Read the model definition and answer for the solid it produces. Units are mm, in the model's axes. A direction names the side the tool comes from. Round coordinates to 2 decimals unless told otherwise and drop trailing zeros. Order: outer loops, then holes, each group sorted by start corner. A loop starts at its lowest first (then second) coordinate and runs counter-clockwise, first axis right, second up. Notation, with made-up numbers: (81.5, 55.25) -> (85.5, 55.25) arc R14 ccw to (85.5, 80.25) -> close; hole circle Ø7 at (69.25, 86.25). An arc over 180 degrees is marked (long way). Use a Markdown table: item, result. Add a question column.
1. Section D-D, the plane z = 11.25 is taken. Give the vertices of the cut face in (x, y).
2. The mould has two halves that part along Y. Classify faces 5 (the face through (11, -4.25, 8)), 6 (the face through (3.73, -3.8, 1.48)), 7 (the face through (0, -5, 8)): +Y half, -Y half, draft (parallel to the pull), parting line (faces both ways), or undercut.
3. Section A-A, the plane x = 8 is taken. Give the vertices of the cut face in (y, z) (3 decimals).
4. Given pin 1 (1.1 mm diameter, centred on x = 4.5, y = -7, fed in from -Z); pin 2 (0.7 mm diameter, centred on x = 13.5, y = -4.5, fed in from -Z); pin 3 (1 mm diameter, centred on y = -9, z = 6, fed in from +X), each flat-ended and moving along its own axis, determine where each tip first touches the part or whether it passes through.
5. Consider L1, parallel to Y at x = 5.14, z = 1.5; L2, parallel to X at y = -7.63, z = 1.6; L3, parallel to Z at x = 16.9, y = -7.64. Determine where each line is inside the solid, lowest interval first. Write a range as [from, to].
6. Section B-B, the plane x = 12.75 is taken. Give the vertices of the cut face in (y, z), then the cut area to 3 significant figures.
7. Section C-C, the plane y = -5.25 is taken. Give the vertices of the cut face in (x, z), then the cut area to 3 significant figures.
8. For faces 1 (the face through (2, -3.7, 10)), 2 (the face through (13, -2, 9.73)), 3 (the face through (1, -3, 1)), 4 (the face through (13, -5, 13.83)), determine the directions among +Z, -Z, +X, -X, +Y, -Y from which every point of the face is accessible in a straight line to the end or side of a thin tool.
```python
from build123d import *

# Parameters (mm, degrees)
F1_DEPTH  = 10.14
F2_R      = 1.91
F2_W      = 1
F2_H      = 2.7
F3_DEPTH  = 3
F4_W      = 2.5
F4_H      = 3.45
F5_DEPTH  = 5
F6_R      = 1.5
F7_DEPTH  = 2
F9_DEPTH  = 8.95
F11_DEPTH = 8.95
F12_R     = 0.75
F13_DEPTH = 5
F14_R     = 0.75
F15_DEPTH = 5
F16_W     = 9.15
F16_H     = 1.7
F17_DEPTH = 1
F20_DEPTH = 1


with BuildPart() as f1:
    # F0 (on Front) → F1 (new body)
    with BuildSketch(Plane.XZ):
        Polygon((8.4, 15), (0, 15), (0, 0), (8.4, 0), (8.4, 9.23), (17.35, 9.23), (17.35, 13.83), (8.4, 13.83), align=None)
    extrude(amount=F1_DEPTH)

    # F2 (on face) → F3 (cut)
    with BuildSketch(Plane(origin=(0, 0, 0), x_dir=(1, 0, 0), z_dir=(0, 0, -1))):
        with Locations((5.14, 2.51)):
            Circle(F2_R)
        with Locations((5.14, 7.63)):
            Circle(F2_R)
        with Locations((1.5, 2.55)):
            Rectangle(F2_W, F2_H)
        with Locations((1.5, 7.59)):
            Rectangle(F2_W, F2_H)
    extrude(amount=-F3_DEPTH, mode=Mode.SUBTRACT)

    # F4 (on face) → F5 (cut)
    with BuildSketch(Plane(origin=(0, 0, 0), x_dir=(0, -1, 0), z_dir=(-1, 0, 0))):
        with Locations((7.69, 10.075)):
            Rectangle(F4_W, F4_H)
        with Locations((2.45, 10.075)):
            Rectangle(F4_W, F4_H)
    extrude(amount=-F5_DEPTH, mode=Mode.SUBTRACT)

    # F6 (on face) → F7 (cut)
    with BuildSketch(Plane.YZ.offset(17.35)):
        with Locations((-2.5, 11.73)):
            Circle(F6_R)
        with Locations((-7.64, 11.73)):
            Circle(F6_R)
    extrude(amount=-F7_DEPTH, mode=Mode.SUBTRACT)

    # F8 (on face) → F9 (cut)
    with BuildSketch(Plane.YZ.offset(17.35)):
        Polygon((-9.2476493944, 9.73), (-9.09, 9.23), (-7.64, 9.23), (-7.64, 9.73), align=None)
        Polygon((-7.64, 9.73), (-7.64, 9.23), (-6.19, 9.23), (-6.0323506056, 9.73), align=None)
        Polygon((-1.05, 9.23), (-0.8923506056, 9.73), (-4.1076493944, 9.73), (-3.95, 9.23), align=None)
    extrude(amount=-F9_DEPTH, mode=Mode.SUBTRACT)

    # F10 (on face) → F11 (join, through all)
    with BuildSketch(Plane.YZ.offset(17.35)):
        with BuildLine():
            Line((-9.5071100664, 13.83), (-5.7728899336, 13.83))
            ThreePointArc((-5.7728899336, 13.83), (-7.64, 14.54), (-9.5071100664, 13.83))
        make_face()
        with BuildLine():
            ThreePointArc((-0.6328899336, 13.83), (-2.5, 14.54), (-4.3671100664, 13.83))
            Line((-4.3671100664, 13.83), (-0.6328899336, 13.83))
        make_face()
    extrude(amount=-F11_DEPTH)

    # F12 (on face) → F13 (cut)
    with BuildSketch(Plane.YZ.offset(15.35)):
        with Locations((-7.64, 11.73)):
            Circle(F12_R)
    extrude(amount=-F13_DEPTH, mode=Mode.SUBTRACT)

    # F14 (on face) → F15 (cut)
    with BuildSketch(Plane.YZ.offset(15.35)):
        with Locations((-2.5, 11.73)):
            Circle(F14_R)
    extrude(amount=-F15_DEPTH, mode=Mode.SUBTRACT)

    # F16 (on face) → F17 (cut)
    with BuildSketch(Plane.YZ.offset(8.4)):
        with Locations((-5.07, 1.85)):
            Rectangle(F16_W, F16_H)
    extrude(amount=-F17_DEPTH, mode=Mode.SUBTRACT)

    # F19 (on offset) → F20 (join)
    with BuildSketch(Plane(origin=(0, -3.25, 0), x_dir=(-1, 0, 0), z_dir=(0, 1, 0))):
        Polygon((-8.4, 6.43), (-8.4, 8.23), (-13.4703818727, 8.23), (-13.803715206, 8.6026779962), (-14.4, 8.0693446629), (-13.4, 6.9513106742), align=None)
    extrude(amount=-F20_DEPTH)


solid = f1.part
```
Verdict:
| question | item | result |
|---|---|---|
| 1 | outline | (0, -10.14) -> (17.35, -10.14) -> (17.35, -9.06) -> (15.35, -9.06) -> (15.35, -8.22) -> (10.35, -8.22) -> (10.35, -7.06) -> (15.35, -7.06) -> (15.35, -6.22) -> (17.35, -6.22) -> (17.35, -3.92) -> (15.35, -3.92) -> (15.35, -3.08) -> (10.35, -3.08) -> (10.35, -1.92) -> (15.35, -1.92) -> (15.35, -1.08) -> (17.35, -1.08) -> (17.35, 0) -> (0, 0) -> (0, -1.2) -> (5, -1.2) -> (5, -3.7) -> (0, -3.7) -> (0, -6.44) -> (5, -6.44) -> (5, -8.94) -> (0, -8.94) -> close |
| 2 | face 5 | -Y half |
| 2 | face 6 | undercut |
| 2 | face 7 | draft |
| 3 | outline | (-10.14, 0) -> (0, 0) -> (0, 15) -> (-10.14, 15) -> close; hole (-9.645, 1) -> (-0.495, 1) -> (-0.495, 2.7) -> (-9.645, 2.7) -> close |
| 4 | pin 1 | stops at z = 3 |
| 4 | pin 2 | stops at z = 6.94 |
| 4 | pin 3 | stops at x = 8.4 |
| 5 | L1 | y = [-10.14, -9.54], [-5.72, -4.42], [-0.6, 0] |
| 5 | L2 | x = [0, 1], [2, 3.23], [7.05, 7.4] |
| 5 | L3 | z = [9.73, 10.23], [13.23, 14.54] |
| 6 | outline | (-10.14, 9.23) -> (-9.09, 9.23) -> (-9.25, 9.73) -> (-6.03, 9.73) -> (-6.19, 9.23) -> (-3.95, 9.23) -> (-4.11, 9.73) -> (-0.89, 9.73) -> (-1.05, 9.23) -> (0, 9.23) -> (0, 13.83) -> (-0.63, 13.83) arc R2.81 ccw to (-4.37, 13.83) -> (-5.77, 13.83) arc R2.81 ccw to (-9.51, 13.83) -> (-10.14, 13.83) -> close; (-4.25, 6.88) -> (-3.25, 6.88) -> (-3.25, 8.23) -> (-4.25, 8.23) -> close; hole circle Ø1.5 at (-7.64, 11.73); hole circle Ø1.5 at (-2.5, 11.73) |
| 6 | area | 45.0 mm2 |
| 7 | outline | (0, 0) -> (8.4, 0) -> (8.4, 1) -> (7.4, 1) -> (7.4, 2.7) -> (8.4, 2.7) -> (8.4, 9.23) -> (17.35, 9.23) -> (17.35, 13.83) -> (8.4, 13.83) -> (8.4, 15) -> (0, 15) -> close |
| 7 | area | 165 mm2 |
| 8 | face 1 | -X |
| 8 | face 2 | +X |
| 8 | face 3 | -Z |
| 8 | face 4 | +Z, +X |
